```python
from build123d import *

# Parameters (mm, degrees)
F0_R     = 7.5
F1_DEPTH = 22
F3_DEPTH = 18
F4_W     = 15
F4_H     = 11.0249955803
F5_DEPTH = 5
F6_DEPTH = 25
F7_DEPTH = 20
F8_W     = 3.414438339
F8_H     = 8.0012119859
F9_DEPTH = 11.0259955803


with BuildPart() as f1:
    # F0 (on Top) → F1 (new body)
    with BuildSketch(Plane.XY):
        Circle(F0_R)
    extrude(amount=F1_DEPTH)

    # F2 (on face) → F3 (cut)
    with BuildSketch(Plane.XY.offset(22)):
        with BuildLine():
            Line((2, -1.5), (2, 1.5))
            ThreePointArc((2, 1.5), (-2.5, 0), (2, -1.5))
        make_face()
    extrude(amount=-F3_DEPTH, mode=Mode.SUBTRACT)

    # F4 (on face) → F5 (join)
    with BuildSketch(Plane(origin=(0, 0, 0), x_dir=(1, 0, 0), z_dir=(0, 0, -1))):
        with BuildLine():
            ThreePointArc((7.5, 0), (0, -7.5), (-7.5, 0))
            Line((-7.5, 0), (-7.5, -12.4750044197))
            Line((-7.5, -12.4750044197), (7.5, -12.4750044197))
            Line((7.5, -12.4750044197), (7.5, 0))
        make_face()
        with Locations((0, -17.9875022098)):
            Rectangle(F4_W, F4_H)
    extrude(amount=-F5_DEPTH)

    # F4 (on face) → F6 (join)
    with BuildSketch(Plane(origin=(0, 0, 0), x_dir=(1, 0, 0), z_dir=(0, 0, -1))):
        with Locations((0, -17.9875022098)):
            Rectangle(F4_W, F4_H)
    extrude(amount=F6_DEPTH)

    # F4 (on face) → F7 (join)
    with BuildSketch(Plane(origin=(0, 0, 0), x_dir=(1, 0, 0), z_dir=(0, 0, -1))):
        with BuildLine():
            Line((-7.5, 12.4750044197), (-7.5, 0))
            ThreePointArc((-7.5, 0), (0, 7.5), (7.5, 0))
            Line((7.5, 0), (7.5, 12.4750044197))
            Line((7.5, 12.4750044197), (-7.5, 12.4750044197))
        make_face()
        with Locations((0, 17.9875022098)):
            Rectangle(F4_W, F4_H)
    extrude(amount=-F7_DEPTH)

    # F8 (on face) → F9 (cut, through all)
    with BuildSketch(Plane.XZ.offset(-12.4750044197)):
        with Locations((3.3099151915, -18.999394007)):
            Rectangle(F8_W, F8_H)
        with Locations((-3.3099151915, -18.999394007)):
            Rectangle(F8_W, F8_H)
    extrude(amount=-F9_DEPTH, mode=Mode.SUBTRACT)


solid = f1.part
```
Can you work these out from the model? Positions are in its coordinate system, mm. A direction names the side the tool comes from. Round coordinates to 2 decimals unless told otherwise and drop trailing zeros. Loops run counter-clockwise (first coordinate to the right, second up) from the corner with the lowest first, then second, coordinate; pieces in that order, holes last.
Item 1: Please list where these lines run through material, in increasing order: L1, parallel to X at y = 0, z = 10; L2, parallel to Y at x = 0, z = 11.25; L3, parallel to Z at x = 3.75, y = -5.5.
Item 2: Suppose I cut it at A-A, the plane y = 18.5. Write out the boundary of the cut face in (x, z).
Item 3: Suppose I cut it at B-B, the plane x = 4. Write out the boundary of the cut face in (y, z) (3 decimals), then the cut area to 3 significant figures.
Item 4: Suppose I cut it at C-C, the plane x = 0. Write out the boundary of the cut face in (y, z) (3 decimals).
Item 5: Suppose I cut it at D-D, the plane z = -5. Write out the boundary of the cut face in (x, y) (3 decimals), then the cut area to 3 significant figures.
Item 6: Will these pins go through, and if not, where does the flat tip stop? pin 1 Ø1 at (x, y) = (-2.5, 20) entering from +Z; pin 2 Ø3 at (x, y) = (0, 0) entering from +Z; pin 3 Ø3 at (x, y) = (-3.5, -14) entering from -Z.
Item 7: If we mould it in two halves opening along Y, with no side actions, what happens to faces 1 (the flat face through (2, 0, 13)), 2 (the flat face through (3, 18, -14.999)), 3 (the flat face through (0, 0, 4)), 4 (the flat face through (0, 23.5, -10))? For each: +Y half, -Y half, draft (parallel to the pull), parting line (faces both ways), or undercut.
Item 8: Which directions (+Z, -Z, +X, -X, +Y, -Y) give clear straight access to the entire face, cutting with the end or side of a thin tool? Please do faces 5 (the flat face through (0, -6, 0)), 6 (the flat face through (-5.017, 18, -19)), 7 (the cylindrical face through (-2.5, 0.1, 13.1)).
Reported:
1. L1: x = -7.5 to -2.5, 2 to 7.5
1. L2: y = -23.5 to -2.5, 2.5 to 7.5
1. L3: z = 0 to 22
2. outline: (-7.5, -25) - (7.5, -25) - (7.5, 5) - (-7.5, 5) - close; hole (-5.02, -23) - (-1.6, -23) - (-1.6, -15) - (-5.02, -15) - close; hole (1.6, -23) - (5.02, -23) - (5.02, -15) - (1.6, -15) - close
3. outline: (-23.5, 0) - (12.475, 0) - (12.475, -14.999) - (23.5, -14.999) - (23.5, 5) - (6.344, 5) - (6.344, 22) - (-6.344, 22) - (-6.344, 20) - (-23.5, 20) - close; (12.475, -25) - (23.5, -25) - (23.5, -23) - (12.475, -23) - close
3. area: 895 mm2
4. outline: (-23.5, 0) - (12.475, 0) - (12.475, -25) - (23.5, -25) - (23.5, 5) - (7.5, 5) - (7.5, 22) - (2.5, 22) - (2.5, 4) - (-2.5, 4) - (-2.5, 22) - (-7.5, 22) - (-7.5, 20) - (-23.5, 20) - close
5. outline: (-7.5, 12.475) - (7.5, 12.475) - (7.5, 23.5) - (-7.5, 23.5) - close
5. area: 165 mm2
6. pin 1: stops at z = 5
6. pin 2: stops at z = 4
6. pin 3: stops at z = 0
7. face 1: undercut
7. face 2: draft
7. face 3: undercut
7. face 4: +Y half
8. face 5: -Z, +X, -X, -Y
8. face 6: +Y, -Y
8. face 7: +Z
